Design review of the part built by this model. Coordinates are the model's own, in mm. Face numbers are marked on the shaded views. A direction names the side the tool comes from. Coordinates: 2 decimals unless noted, no trailing zeros. Write each loop counter-clockwise with the first axis right and the second up, starting at its lowest first coordinate (ties: lowest second). Pieces come first, ordered by that corner, then holes.
Q1. Add section D-D, the plane z = -6.5. Give the boundary of the cut face in (x, y), plus the area to 3 significant figures.
Q2. Add section C-C, the plane x = 1.5. Give the boundary of the cut face in (y, z), plus the area to 3 significant figures.
Q3. Add section B-B, the plane y = -1.5. Give the boundary of the cut face in (x, z).
Q4. Add section A-A, the plane z = 0. Give the boundary of the cut face in (x, y), plus the area to 3 significant figures.
Q5. Clearance check with flat-ended pins moving along their axes: pin 1 Ø0.8 at (y, z) = (4.5, -2) entering from -X; pin 2 Ø6 at (x, z) = (5.5, -5.5) entering from -Y; pin 3 Ø1 at (x, z) = (-6, 2) entering from +Y. State where each tip first meets the part, or that it passes through.
Q6. The part is to be moulded in two halves that separate along Y. For the marked faces 1, 2, 3 and 4, say which applies: +Y half, -Y half, draft (parallel to the pull), parting line (faces both ways), or undercut.
Q7. To check wall thickness, follow probe 1 along Y at (x, z) = (-3, -4.25); probe 2 along Z at (x, y) = (-1.5, 2.5); probe 3 along Z at (x, y) = (0.25, 1). State the ranges of each line that lie inside material, in increasing order.
Q8. Machinability: for the marked faces 5, 6 and 7, which of the approach directions +Z, -Z, +X, -X, +Y, -Y give a long, thin tool a straight path to every point of the face, cutting with its end or side? Answer none if there is none.
from build123d import *

# Parameters (mm, degrees)
EXTRUDE_1_DEPTH      = 10
EXTRUDE_1_DEPTH_BACK = 8
SKETCH_2_R           = 2
CUT_EXTRUDE_1_DEPTH  = 6.3
EXTRUDE_2_DEPTH      = 18
CUT_EXTRUDE_2_DEPTH  = 4
SKETCH_5_W           = 0.05
SKETCH_5_H           = 18
CUT_EXTRUDE_3_DEPTH  = 1
FILLET_1_R           = 1


with BuildPart() as part:
    # Эскиз1 → Бобышка-Вытянуть1 (new body, two sides)
    with BuildSketch(Plane.XY) as extrude_1_sk:
        with BuildLine():
            Line((3.505219116, 0), (-3.505219116, 0))
            ThreePointArc((-3.505219116, 0), (-3.948686522, 0.1037095), (-4.300170362, 0.393326681))
            Line((-4.300170362, 0.393326681), (-6.9, 3.8))
            Line((-6.9, 3.8), (-4.85, 3.8))
            Line((-4.85, 3.8), (-4.85, 5.3))
            Line((-4.85, 5.3), (4.85, 5.3))
            Line((4.85, 5.3), (4.85, 3.8))
            Line((4.85, 3.8), (6.9, 3.8))
            Line((6.9, 3.8), (4.300170362, 0.393326681))
            ThreePointArc((4.300170362, 0.393326681), (3.948686522, 0.1037095), (3.505219116, 0))
        make_face()
    extrude(amount=EXTRUDE_1_DEPTH)
    extrude(extrude_1_sk.sketch, amount=-EXTRUDE_1_DEPTH_BACK)

    # Эскиз2 → Вырез-Вытянуть1 (cut, through all)
    with BuildSketch(Plane(origin=(0, 5.3, 0), x_dir=(1, 0, 0), z_dir=(0, 1, 0))):
        with Locations(Location((0, 0, 0), (0, 0, 270))):  # turned: the seam where the file's is
            Circle(SKETCH_2_R)
    extrude(amount=-CUT_EXTRUDE_1_DEPTH, mode=Mode.SUBTRACT)

    # Эскиз3 → Бобышка-Вытянуть2 (add)
    with BuildSketch(Plane.XY.offset(10)):
        with BuildLine():
            Line((6.9, 3.8), (1.924195295, -2.720019958))
            ThreePointArc((1.924195295, -2.720019958), (0.869743776, -3.588871499), (-0.460658443, -3.9))
            Line((-0.460658443, -3.9), (-2.630413016, -3.9))
            ThreePointArc((-2.630413016, -3.9), (-2.680413016, -3.95), (-2.630413016, -4))
            Line((-2.630413016, -4), (-0.460658443, -4))
            ThreePointArc((-0.460658443, -4), (0.914090516, -3.678500549), (2.00369042, -2.78068729))
            Line((2.00369042, -2.78068729), (6.979495125, 3.739332668))
            ThreePointArc((6.979495125, 3.739332668), (6.970081228, 3.809413896), (6.9, 3.8))
        make_face()
    extrude(amount=-EXTRUDE_2_DEPTH)

    # Эскиз4 → Вырез-Вытянуть2 (cut)
    with BuildSketch(Plane.XZ.offset(4)):
        with BuildLine():
            Line((0, 4.5), (-4.5, 4.5))
            Line((-4.5, 4.5), (-4.5, 0))
            Line((-4.5, 0), (-4.5, -4.5))
            Line((-4.5, -4.5), (0, -4.5))
            ThreePointArc((0, -4.5), (4.5, 0), (0, 4.5))
        make_face()
    extrude(amount=-CUT_EXTRUDE_2_DEPTH, mode=Mode.SUBTRACT)

    # Эскиз5 → Вырез-Вытянуть3 (cut)
    with BuildSketch(Plane.XZ.offset(4)):
        with Locations((-2.655413016, 1)):
            Rectangle(SKETCH_5_W, SKETCH_5_H)
    extrude(amount=-CUT_EXTRUDE_3_DEPTH, mode=Mode.SUBTRACT)

    # Скругление1
    fillet_1_edges = [part.edges().sort_by_distance(p)[0] for p in [
        (-2.630413016, -3.95, 4.5),
        (-2.630413016, -3.95, -4.5),
        (-2.630413016, -3.95, 10),
        (-2.630413016, -3.95, -8),
    ]]
    fillet(fillet_1_edges, radius=FILLET_1_R)


solid = part.part
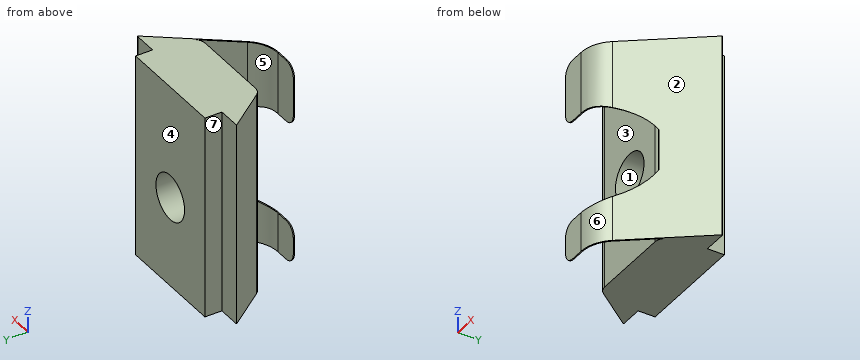
Here are the results:
1. outline: (-6.9, 3.8) - (-4.3, 0.39) arc R1 ccw to (-3.51, 0) - (3.51, 0) arc R1 ccw to (4.3, 0.39) - (1.92, -2.72) arc R3 cw to (-0.46, -3.9) - (-2.63, -3.9) - (-2.63, -4) - (-0.46, -4) arc R3.1 ccw to (2, -2.78) - (6.98, 3.74) arc R0.05 ccw to (6.9, 3.8) - (4.85, 3.8) - (4.85, 5.3) - (-4.85, 5.3) - (-4.85, 3.8) - close
1. area: 57.2 mm2
2. outline: (-3.3, -8) - (-3.17, -8) - (-3.17, -4.24) - (-3.3, -4.24) - close; (-3.3, 4.24) - (-3.17, 4.24) - (-3.17, 10) - (-3.3, 10) - close; (0, -8) - (5.3, -8) - (5.3, -1.32) - (0, -1.32) - close; (0, 1.32) - (5.3, 1.32) - (5.3, 10) - (0, 10) - close
2. area: 82.6 mm2
3. outline: (2.86, -8) - (2.98, -8) - (2.98, -3.37) arc R4.5 cw to (2.86, -3.48) - close; (2.86, 3.48) arc R4.5 cw to (2.98, 3.37) - (2.98, 10) - (2.86, 10) - close
4. outline: (-6.9, 3.8) - (-4.3, 0.39) arc R1 ccw to (-3.51, 0) - (-2, 0) - (-2, 5.3) - (-4.85, 5.3) - (-4.85, 3.8) - close; (2, 0) - (3.51, 0) arc R1 ccw to (4.3, 0.39) - (4, 0) - (4.13, 0) - (6.98, 3.74) arc R0.05 ccw to (6.9, 3.8) - (4.85, 3.8) - (4.85, 5.3) - (2, 5.3) - close
4. area: 35.2 mm2
5. pin 1: stops at x = -4.85
5. pin 2: stops at y = -2.13
5. pin 3: stops at y = 3.8
6. face 1: draft
6. face 2: -Y half
6. face 3: undercut
6. face 4: +Y half
7. probe 1: y = 0 to 5.3
7. probe 2: z = -8 to -1.32, 1.32 to 10
7. probe 3: z = -8 to -1.98, 1.98 to 10
8. face 5: +Z, -Z, -X
8. face 6: +Z, -Z, +X, -Y
8. face 7: +Z, -Z, -X, +Y
